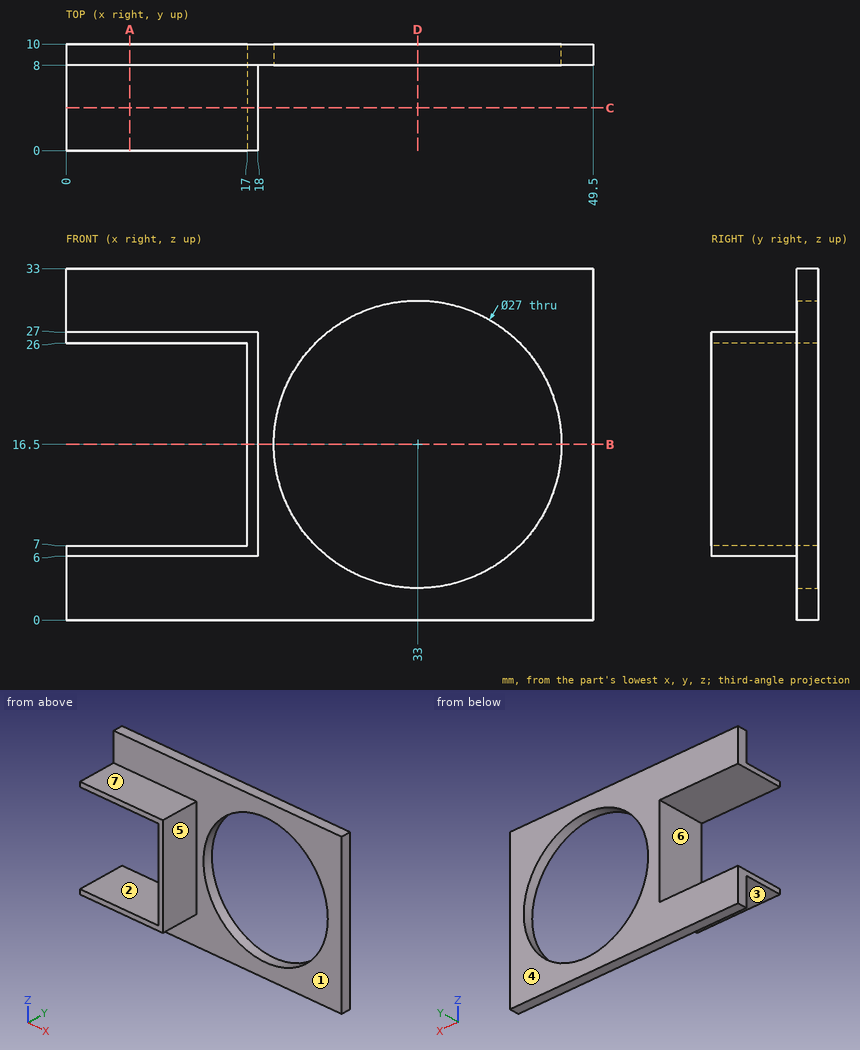
Job drawing, mm, ordinate dimensions from the low corner. One solid piece. A direction names the side the tool comes from. Coordinates: 2 decimals unless noted, no trailing zeros. Order: outer loops, then holes, each group sorted by start corner. A loop starts at its lowest first (then second) coordinate and runs counter-clockwise, first axis right, second up. Notation, with made-up numbers: M -19.75,41.25 L 25.25,41.25 A20 ccw 25.25,76.25 Z; hole C -7,-9.75 d11. An arc over 180 degrees is marked long. One line per question, with ' | ' between items.
Q1. Slice it at D-D (x = 33). Give the cut face in (y, z).
A:
outline: M 8,0 L 10,0 L 10,3 L 8,3 Z; M 8,30 L 10,30 L 10,33 L 8,33 Z
Q2. Slice it at B-B (z = 16.5). Give the cut face in (x, y).
A:
outline: M 17,0 L 18,0 L 18,8 L 19.5,8 L 19.5,10 L 17,10 Z; M 46.5,8 L 49.5,8 L 49.5,10 L 46.5,10 Z
Q3. Slice it at A-A (x = 6). Give the cut face in (y, z), and give its area (3 significant figures).
A:
outline: M 0,6 L 8,6 L 8,0 L 10,0 L 10,7 L 0,7 Z; M 0,26 L 10,26 L 10,33 L 8,33 L 8,27 L 0,27 Z | area: 44.0 mm^2
Q4. Pin check, flat tips, straight feed: P1, Ø6, axis at x = 11.5, y = 2.5, coming from the +Z side; P2, Ø4, axis at x = 6, y = 5, coming from the -Z side. Stop position of each tip, or through.
A:
P1: stops at z = 27 | P2: stops at z = 6
Q5. Slice it at C-C (y = 4). Give the cut face in (x, z).
A:
outline: M 0,6 L 18,6 L 18,27 L 0,27 L 0,26 L 17,26 L 17,7 L 0,7 Z
Q6. Two-plate mould, pull along Z, no slides. Class the marked faces 1, 2 and 3: +Z half, -Z half, draft (parallel to the pull), parting line (faces both ways), or undercut.
A:
face 1: draft | face 2: undercut | face 3: -Z half
Q7. Drill centre lines: line 1 (Z direction, x = 33, y = 8.5); line 2 (Z direction, x = 14, y = 4.5); line 3 (Y direction, x = 6, z = 30.5). Where is each one in solid material? Low to high.
A:
line 1: z = 0 to 3, 30 to 33 | line 2: z = 6 to 7, 26 to 27 | line 3: y = 8 to 10
Q8. 3-axis set-ups, long thin cutter, end or side, ignore diameter. For the marked faces 4, 5, 6 and 7: which of +Z, -Z, +X, -X, +Y, -Y reach the whole face in a straight line?
A:
face 4: +Z, -Z, +X, -X, +Y | face 5: +Z, -Z, +X, -Y | face 6: -X, +Y, -Y | face 7: +Z, +X, -X, -Y
